Part print with two shaded views. Sizes in mm from the minimum x, y, z corner. Round coordinates to 2 decimals unless told otherwise and drop trailing zeros. Loops run counter-clockwise (first coordinate to the right, second up) from the corner with the lowest first, then second, coordinate; pieces in that order, holes last. Notation, with made-up numbers: (-5, 24.25) - (30, 24.25) arc R22 cw to (30, 47.25) - close; hole circle Ø9 at (33, 31). An arc over 180 degrees is marked (long way). Use a Markdown table: item, result.
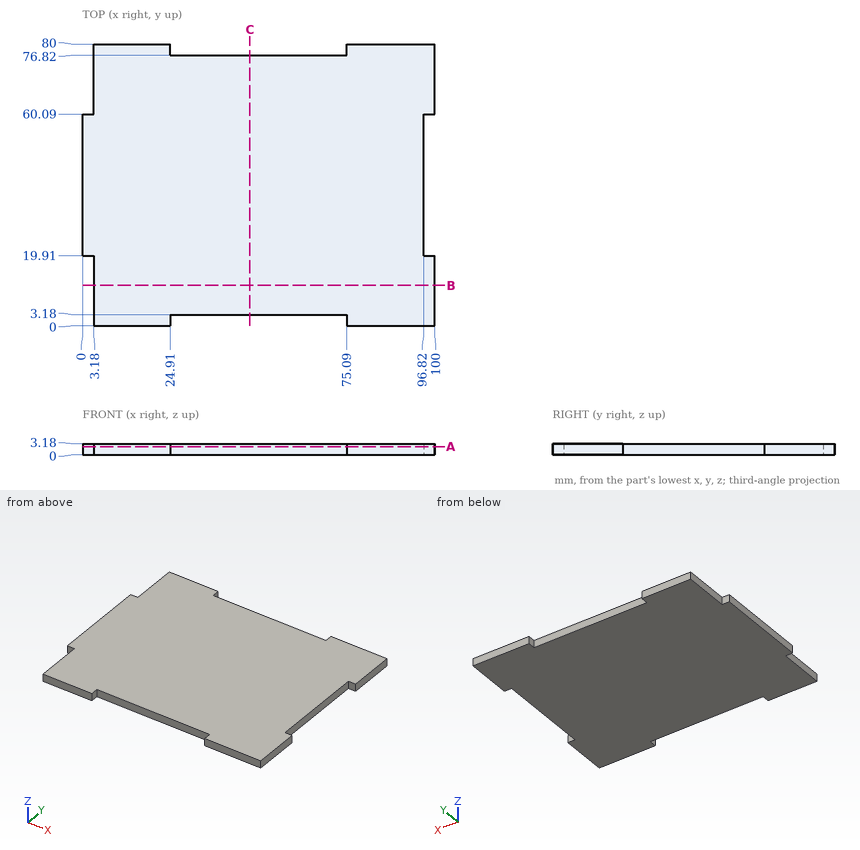
Q1. Cut at A-A, the plane z = 2.35. List the corners of the cut face in (x, y), plus the area to 3 significant figures.
Results found:
| item | result |
|---|---|
| outline | (0, 19.91) - (3.18, 19.91) - (3.18, 0) - (24.91, 0) - (24.91, 3.18) - (75.09, 3.18) - (75.09, 0) - (100, 0) - (100, 19.91) - (96.82, 19.91) - (96.82, 60.09) - (100, 60.09) - (100, 80) - (75.09, 80) - (75.09, 76.82) - (24.91, 76.82) - (24.91, 80) - (3.18, 80) - (3.18, 60.09) - (0, 60.09) - close |
| area | 7,430 mm2 |
Q2. Cut at B-B, the plane y = 11.5. List the corners of the cut face in (x, z), plus the area to 3 significant figures.
Results found:
| item | result |
|---|---|
| outline | (3.18, 0) - (100, 0) - (100, 3.18) - (3.18, 3.18) - close |
| area | 308 mm2 |
Q3. Cut at C-C, the plane x = 47.5. List the corners of the cut face in (y, z), plus the area to 3 significant figures.
Results found:
| item | result |
|---|---|
| outline | (3.18, 0) - (76.82, 0) - (76.82, 3.18) - (3.18, 3.18) - close |
| area | 234 mm2 |
Q4. Drop flat-ended pins along their axis: pin 1 (1 mm diameter, centred on y = 10.5, z = 2, fed in from -X); pin 2 (1 mm diameter, centred on x = 40, z = 2.5, fed in from -Y); pin 3 (1 mm diameter, centred on x = 1, z = 1, fed in from +Y). Give the stop position or say it passes through.
Results found:
| item | result |
|---|---|
| pin 1 | stops at x = 3.18 |
| pin 2 | stops at y = 3.18 |
| pin 3 | stops at y = 60.09 |
Q5. Probe line 1 (X direction, y = 49, z = 1.15); line 2 (X direction, y = 7, z = 1); line 3 (Y direction, x = 45.5, z = 1.85). List the from-to ranges inside material, lowest first.
Results found:
| item | result |
|---|---|
| line 1 | x = 0 to 96.82 |
| line 2 | x = 3.18 to 100 |
| line 3 | y = 3.18 to 76.82 |
